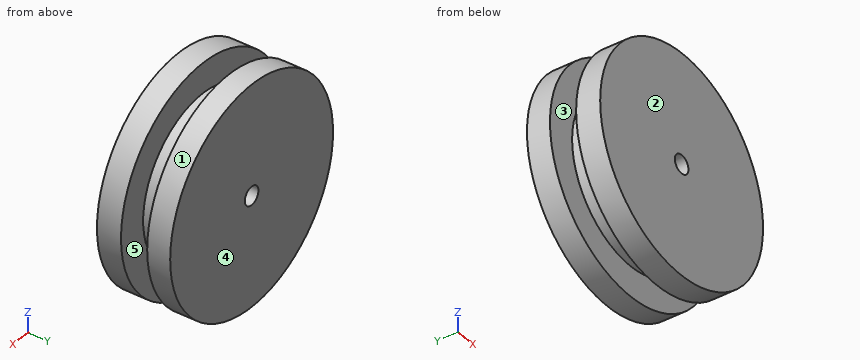
```python
from build123d import *

# Parameters (mm, degrees)
F0_R     = 38.1
F1_DEPTH = 12.7
F2_W     = 20.0255792588
F2_H     = 9.0756523423
F4_R     = 3.175
F5_DEPTH = 25.401


with BuildPart() as f1:
    # F0 (on Front) → F1 (new body, symmetric)
    with BuildSketch(Plane.XZ):
        Circle(F0_R)
    extrude(amount=F1_DEPTH, both=True)

    # F2 (on Top) → F3 (revolve, cut)
    with BuildSketch(Plane.XY):
        with Locations((-37.7547862008, 0.1815122087)):
            Rectangle(F2_W, F2_H)
    revolve(axis=Axis((0, -0.3630269784, 0), (0, -1, 0)), mode=Mode.SUBTRACT)

    # F4 (on face) → F5 (cut, through all)
    with BuildSketch(Plane.XZ.offset(12.7)):
        Circle(F4_R)
    extrude(amount=-F5_DEPTH, mode=Mode.SUBTRACT)


solid = f1.part
```
For this review, take the finished solid that the model builds, in its own axes (mm). Face numbers are marked on the shaded views. A direction names the side the tool comes from. Coordinates: 2 decimals unless noted, no trailing zeros. Write each loop counter-clockwise with the first axis right and the second up, starting at its lowest first coordinate (ties: lowest second). Pieces come first, ordered by that corner, then holes. Notation, with made-up numbers: (37, 81.25) -> (43, 81.25) arc R38 cw to (43, 119.25) -> close; hole circle Ø6 at (-15, 59.5). An arc over 180 degrees is marked (long way). Put each result on its own line as item: value.
Q1. Wall thickness on L1, parallel to Z at x = 0, y = 5.75 (3 decimals); L2, parallel to Z at x = 0, y = -3.75 (3 decimals); L3, parallel to Y at x = -27.5, z = -12: over which ranges is each line inside the solid? List them lowest first.
From the geometry:
L1: z = -38.1 to -3.175, 3.175 to 38.1
L2: z = -27.742 to -3.175, 3.175 to 27.742
L3: y = -12.7 to -4.36, 4.72 to 12.7
Q2. Take a section at D-D, the plane z = 29. State the section outline as (x, y) points.
From the geometry:
outline: (-24.71, -12.7) -> (24.71, -12.7) -> (24.71, -4.36) -> (-24.71, -4.36) -> close; (-24.71, 4.72) -> (24.71, 4.72) -> (24.71, 12.7) -> (-24.71, 12.7) -> close
Q3. Take a section at C-C, the plane y = -0.5. State the section outline as (x, z) points (3 decimals), then the cut area to 3 significant figures.
From the geometry:
outline: circle Ø55.484 at (0, 0); hole circle Ø6.35 at (0, 0)
area: 2,390 mm2
Q4. Take a section at B-B, the plane z = 0. State the section outline as (x, y) points (3 decimals).
From the geometry:
outline: (-38.1, -12.7) -> (-3.175, -12.7) -> (-3.175, 12.7) -> (-38.1, 12.7) -> (-38.1, 4.719) -> (-27.742, 4.719) -> (-27.742, -4.356) -> (-38.1, -4.356) -> close; (3.175, -12.7) -> (38.1, -12.7) -> (38.1, -4.356) -> (27.742, -4.356) -> (27.742, 4.719) -> (38.1, 4.719) -> (38.1, 12.7) -> (3.175, 12.7) -> close
Q5. Tool access review of the marked faces 4 and 5: name each direction out of +Z, -Z, +X, -X, +Y, -Y from which nothing blocks a thin tool from reaching the whole face with its end or side.
From the geometry:
face 4: +Z, -Z, +X, -X, +Y
face 5: none
Q6. The part is to be moulded in two halves that separate along Y. For the marked faces 1, 2 and 3, say which applies: +Y half, -Y half, draft (parallel to the pull), parting line (faces both ways), or undercut.
From the geometry:
face 1: draft
face 2: -Y half
face 3: undercut
Q7. Clearance check with flat-ended pins moving along their axes: pin 1 Ø1.5 at (y, z) = (2.5, -2.5) entering from -X; pin 2 Ø10 at (y, z) = (7, -16) entering from -X; pin 3 Ø10 at (x, y) = (-1.5, -6) entering from -Z; pin 4 Ø5 at (x, z) = (0, 0) entering from -Y. State where each tip first meets the part, or that it passes through.
From the geometry:
pin 1: stops at x = -27.69
pin 2: stops at x = -36.48
pin 3: stops at z = -38.1
pin 4: passes through
Q8. Take a section at A-A, the plane x = 0. State the section outline as (y, z) points (3 decimals).
From the geometry:
outline: (-12.7, -38.1) -> (-4.356, -38.1) -> (-4.356, -27.742) -> (4.719, -27.742) -> (4.719, -38.1) -> (12.7, -38.1) -> (12.7, -3.175) -> (-12.7, -3.175) -> close; (-12.7, 3.175) -> (12.7, 3.175) -> (12.7, 38.1) -> (4.719, 38.1) -> (4.719, 27.742) -> (-4.356, 27.742) -> (-4.356, 38.1) -> (-12.7, 38.1) -> close
